Geometry: see drawing. Coordinates: mm, zero at the bounding-box minimum. A direction names the side the tool comes from. Give positions to 0.01 mm unless a question says otherwise; leave off trailing zeros. Write each loop counter-clockwise with the first axis right and the second up, starting at its lowest first coordinate (ties: lowest second). Pieces come first, ordered by that corner, then holes. Notation, with made-up numbers: M -38,72 L -10,72 A31 ccw -10,102 Z; hole C -15.75,53 d8. An arc over 180 degrees is marked long. Use CSV: the item, a comma, the result in double quotes. Start each with the question number.
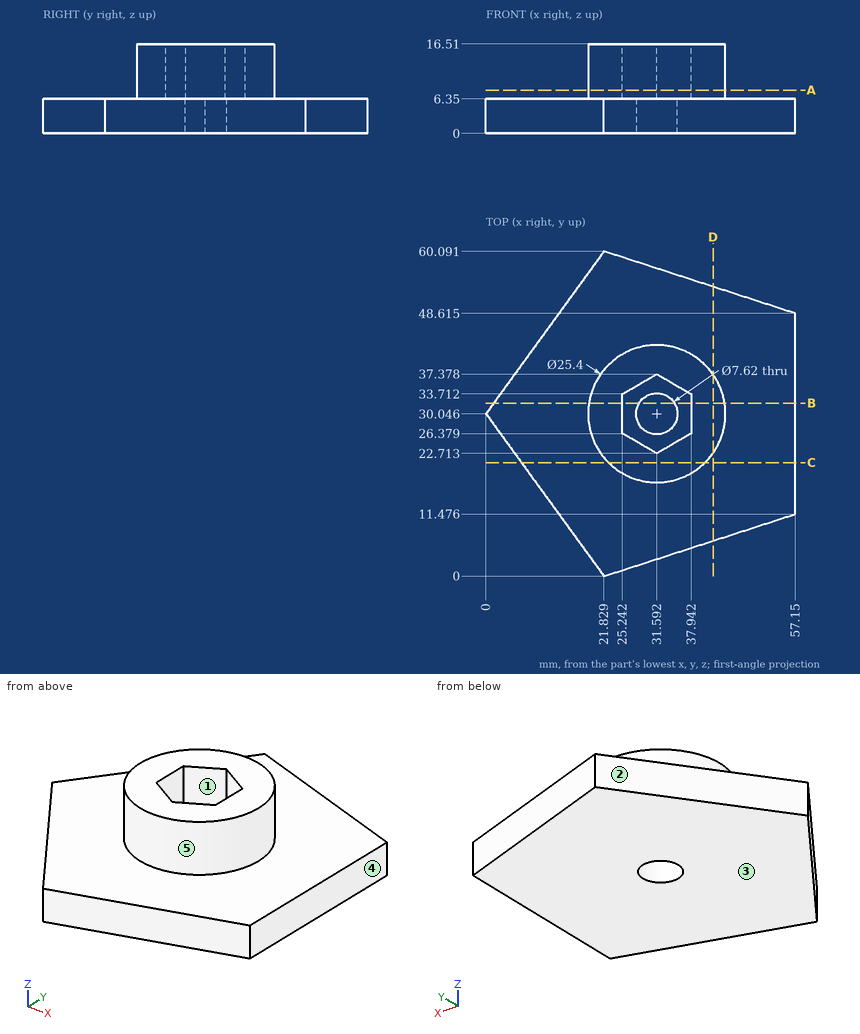
1. Section A-A on z = 8. Return loops of the section in (x, y) (1 decimal).
2. Access query for the marked faces 4 and 5. Directions: +Z, -Z, +X, -X, +Y, -Y. A direction counts if a zero-diameter tool reaches every point of the face in a straight line with its end or side. Return the directions, or none.
3. Pull-direction query (X, two-part tool) for the marked faces 1, 2 and 3; classes: released by +X, released by -X, zero draft, split by the parting line, or undercut.
4. Section C-C on y = 21. Return loops of the section in (x, z).
5. Section B-B on y = 32. Return loops of the section in (x, z).
6. Line query: probe 1 along Y at (x, z) = (32, 15.5); probe 2 along Z at (x, y) = (26.5, 42); probe 3 along X at (y, z) = (24, 14) (1 decimal). Output: solid intervals per line, ascending.
7. First-contact query: pin 1 (3 mm diameter, centred on y = 50, z = 4.5, fed in from -X); pin 2 (3 mm diameter, centred on x = 32.5, z = 8, fed in from +Y); pin 3 (2 mm diameter, centred on y = 31.5, z = 12, fed in from +X). Flat tips, straight axial feed; report the tip coordinate or a pass-through.
8. Section D-D on x = 42. Return loops of the section in (y, z), then the cut area to 3 significant figures.
Resolved:
1,outline,"C 31.6,30 d25.4; hole M 25.2,26.4 L 31.6,22.7 L 37.9,26.4 L 37.9,33.7 L 31.6,37.4 L 25.2,33.7 Z"
2,face 4,"+Z, -Z, +X, +Y, -Y"
2,face 5,"+Z"
3,face 1,"undercut"
3,face 2,"released by -X"
3,face 3,"zero draft"
4,outline,"M 6.57,0 L 57.15,0 L 57.15,6.35 L 40.51,6.35 L 40.51,16.51 L 22.68,16.51 L 22.68,6.35 L 6.57,6.35 Z"
5,outline,"M 1.42,0 L 28.32,0 L 28.32,6.35 L 25.24,6.35 L 25.24,16.51 L 19.04,16.51 L 19.04,6.35 L 1.42,6.35 Z; M 34.86,0 L 57.15,0 L 57.15,6.35 L 44.14,6.35 L 44.14,16.51 L 37.94,16.51 L 37.94,6.35 L 34.86,6.35 Z"
6,probe 1,"y = 17.35 to 22.95, 37.14 to 42.74"
6,probe 2,"z = 0 to 6.35"
6,probe 3,"x = 20.4 to 29.4, 33.8 to 42.8"
7,pin 1,"stops at x = 13.41"
7,pin 2,"stops at y = 42.75"
7,pin 3,"stops at x = 44.28"
8,outline,"M 6.55,0 L 53.54,0 L 53.54,6.35 L 37.32,6.35 L 37.32,16.51 L 22.77,16.51 L 22.77,6.35 L 6.55,6.35 Z"
8,area,"446 mm2"
